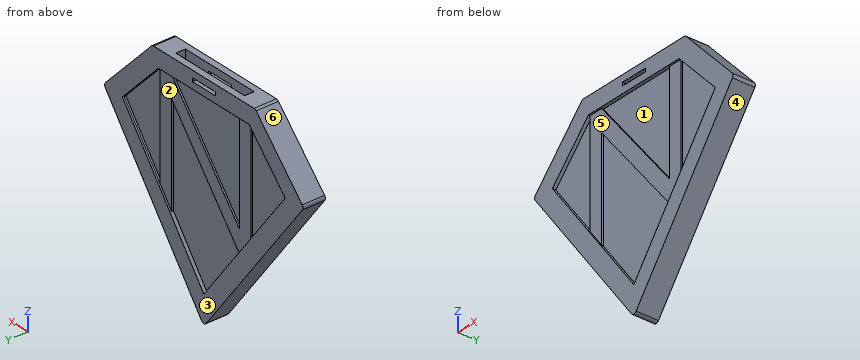
from build123d import *

# Parameters (mm, degrees)
F1_DEPTH  = 3.25
F3_DEPTH  = 0.5
F5_DEPTH  = 0.5
F7_DEPTH  = 0.5
F9_DEPTH  = 0.5
F10_W     = 24
F10_H     = 2.8
F11_DEPTH = 20
F13_DEPTH = 1.4
F14_W     = 8
F14_H     = 1
F15_DEPTH = 25
F16_R     = 1


# Not quite as in the source:
# - ends of sketch curves that miss each other by under 0.0002 mm in the source are joined


with BuildPart() as f1:
    # F0 (on Front) → F1 (new body, symmetric)
    with BuildSketch(Plane.XZ):
        Polygon((18, 18), (0, 18), (-18, 18), (-35, 0), (0, -47), (35, 0), align=None)
    extrude(amount=F1_DEPTH, both=True)

    # F2 (on face) → F3 (cut)
    with BuildSketch(Plane.XZ.offset(3.25)):
        Polygon((15.8447675538, 13), (-15.8447675538, 13), (-28.4822773709, -0.3808927475), (1.162e-07, -38.628522516), (28.4822775009, -0.3808928851), align=None)
    extrude(amount=-F3_DEPTH, mode=Mode.SUBTRACT)

    # F4 (on face) → F5 (cut)
    with BuildSketch(Plane(origin=(0, 3.25, 0), x_dir=(-1, 0, 0), z_dir=(0, 1, 0))):
        Polygon((28.482277527, -0.3808925379), (15.8447676545, 13.0000002682), (-15.8447670441, 13.0000002682), (-28.4822772579, -0.3808928993), (0, -38.6285223599), align=None)
    extrude(amount=-F5_DEPTH, mode=Mode.SUBTRACT)

    # F6 (on face) → F7 (cut)
    with BuildSketch(Plane.XZ.offset(2.75)):
        Polygon((-15.8447675538, -17.3512630734), (-15.8447675538, 13), (-28.4822773709, -0.3808927475), align=None)
        Polygon((28.4822775009, -0.3808928851), (15.8447675538, 13), (15.8447675538, -17.3512633855), align=None)
        Polygon((11.8447675538, -22.7226919569), (-11.8447675538, 6.6308805462), (-11.8447675538, -22.7226916448), (1.162e-07, -38.628522516), align=None)
        Polygon((11.8447675538, -16.3535725031), (11.8447675538, 13), (-11.8447675538, 13), align=None)
    extrude(amount=-F7_DEPTH, mode=Mode.SUBTRACT)

    # F8 (on face) → F9 (cut)
    with BuildSketch(Plane(origin=(0, 2.75, 0), x_dir=(-1, 0, 0), z_dir=(0, 1, 0))):
        Polygon((-15.8447675538, -17.3512633855), (-15.8447675538, 13), (-28.4822772579, -0.3808928993), align=None)
        Polygon((28.482277527, -0.3808925379), (15.8447676545, 13.0000002682), (15.8447675538, -17.3512630734), align=None)
        Polygon((11.8447675538, -16.353572196), (11.8447675538, 13.0000002682), (-11.8447675538, 13.0000002682), align=None)
        Polygon((0, -38.6285223599), (11.8447675538, -22.7226916448), (-11.8447675538, 6.6308808195), (-11.8447675538, -22.7226916448), align=None)
    extrude(amount=-F9_DEPTH, mode=Mode.SUBTRACT)

    # F10 (on face) → F11 (cut)
    with BuildSketch(Plane.XY.offset(18)):
        Rectangle(F10_W, F10_H)
    extrude(amount=-F11_DEPTH, mode=Mode.SUBTRACT)

    # F12 (on Front) → F13 (cut, symmetric)
    with BuildSketch(Plane.XZ):
        with BuildLine():
            Line((12, -2), (-12, -2))
            ThreePointArc((-12, -2), (0, -14), (12, -2))
        make_face()
    extrude(amount=F13_DEPTH, both=True, mode=Mode.SUBTRACT)

    # F14 (on face) → F15 (cut)
    with BuildSketch(Plane.XZ.offset(3.25)):
        with Locations((0, 15.5)):
            Rectangle(F14_W, F14_H)
    extrude(amount=-F15_DEPTH, mode=Mode.SUBTRACT)

    # F16
    f16_edges = [f1.edges().sort_by_distance(p)[0] for p in [
        (0, 0, -47),
        (35, 0, 0),
        (-35, 0, 0),
        (-18, 0, 18),
        (18, 0, 18),
    ]]
    fillet(f16_edges, radius=F16_R)


solid = f1.part
Read the model definition and answer for the solid it produces. Units are mm, in the model's axes. Face numbers are marked on the shaded views. A direction names the side the tool comes from. Round coordinates to 2 decimals unless told otherwise and drop trailing zeros. Write each loop counter-clockwise with the first axis right and the second up, starting at its lowest first coordinate (ties: lowest second). Pieces come first, ordered by that corner, then holes. Notation, with made-up numbers: M 46,43 L 95,43 A20 cw 95,80 Z; hole C 0,26.25 d5. An arc over 180 degrees is marked long. Use a Markdown table: item, result.
1) The part is cut by section A-A (x = -3). Give the number of separate pieces and of enclosed holes in the cut face, plus the area to 3 significant figures.
Answers follow:
| item | result |
|---|---|
| separate pieces | 3 |
| enclosed holes | 0 |
| area | 215 mm2 |
2) The part is cut by section D-D (x = 26). Write down the section's boundary in (y, z).
Answers follow:
| item | result |
|---|---|
| outline | M -3.25,-12.09 L 3.25,-12.09 L 3.25,-3.71 L 2.25,-3.71 L 2.25,2.25 L 3.25,2.25 L 3.25,9.53 L -3.25,9.53 L -3.25,2.25 L -2.25,2.25 L -2.25,-3.71 L -3.25,-3.71 Z |
3) A tool of negligible diameter and unlimited length cuts with its end or side. For the marked faces 1, 2 and 3, from which of +Z, -Z, +X, -X, +Y, -Y can it reach the whole face along a straight path? Write none if from no direction.
Answers follow:
| item | result |
|---|---|
| face 1 | -Y |
| face 2 | +Y |
| face 3 | +Z, -Z, +X, -X, +Y |
4) Straight lines are drawn through the part: line 1 along Z through (x, y) = (1, -2.5) (3 decimals); line 2 along X through (y, z) = (2.5, -13); line 3 along Z through (x, y) = (7, -2.5). For each, find the intervals that lie inside material, in ascending order. Write a range as [from, to].
Answers follow:
| item | result |
|---|---|
| line 1 | z = [-45.657, -37.286], [-9.285, -2.916], [13, 15], [16, 18] |
| line 2 | x = [-25.32, -19.09], [-15.84, -11.84], [-9.14, -4], [11.84, 15.84], [19.09, 25.32] |
| line 3 | z = [-37.6, -29.23], [-16.72, -10.35], [13, 18] |
5) For a pull along X with two mould halves and no side action, classify the marked faces 4, 5 and 6 as pulls with the +X half, pulls with the -X half, needs draft (parallel to the pull), parting line crosses it, or undercut.
Answers follow:
| item | result |
|---|---|
| face 4 | pulls with the +X half |
| face 5 | undercut |
| face 6 | pulls with the -X half |
6) Flat-ended cylindrical pins translate along their axes: pin 1 (7 mm diameter, centred on x = 2, z = -19, fed in from -Y); pin 2 (2 mm diameter, centred on x = 9, z = 0.5, fed in from +Y); pin 3 (3 mm diameter, centred on x = -6, y = 2, fed in from -Z); pin 4 (14 mm diameter, centred on x = 24.5, z = -2, fed in from +Y). Find the tip coordinate at first contact, or state that the pin passes through.
Answers follow:
| item | result |
|---|---|
| pin 1 | stops at y = -2.25 |
| pin 2 | stops at y = 2.25 |
| pin 3 | stops at z = -40.96 |
| pin 4 | stops at y = 3.25 |
7) The part is cut by section C-C (y = -0.25). Write down the section's boundary in (x, z), plus the area to 3 significant figures.
Answers follow:
| item | result |
|---|---|
| outline | M -34.5,-0.67 L -0.8,-45.92 A1 ccw 0.8,-45.92 L 34.5,-0.67 A1 ccw 34.42,0.61 L 18.3,17.69 A1 ccw 17.57,18 L 12,18 L 12,-2 A12 cw -12,-2 L -12,18 L -17.57,18 A1 ccw -18.3,17.69 L -34.42,0.61 A1 ccw Z |
| area | 1,890 mm2 |
